Study the drawing (mm; zero at the part's minimum x, y, z) and answer. A direction names the side the tool comes from. Coordinates: 2 decimals unless noted, no trailing zeros. Loops run counter-clockwise (first coordinate to the right, second up) from the corner with the lowest first, then second, coordinate; pieces in that order, holes last. Notation, with made-up numbers: (-26.75, -5) - (-9.75, -5) arc R24 ccw to (-9.75, 28) - close; hole circle Ø3 at (87.5, 3.5). An arc over 180 degrees is marked (long way). Use CSV: the item, a comma, the result in double quotes.
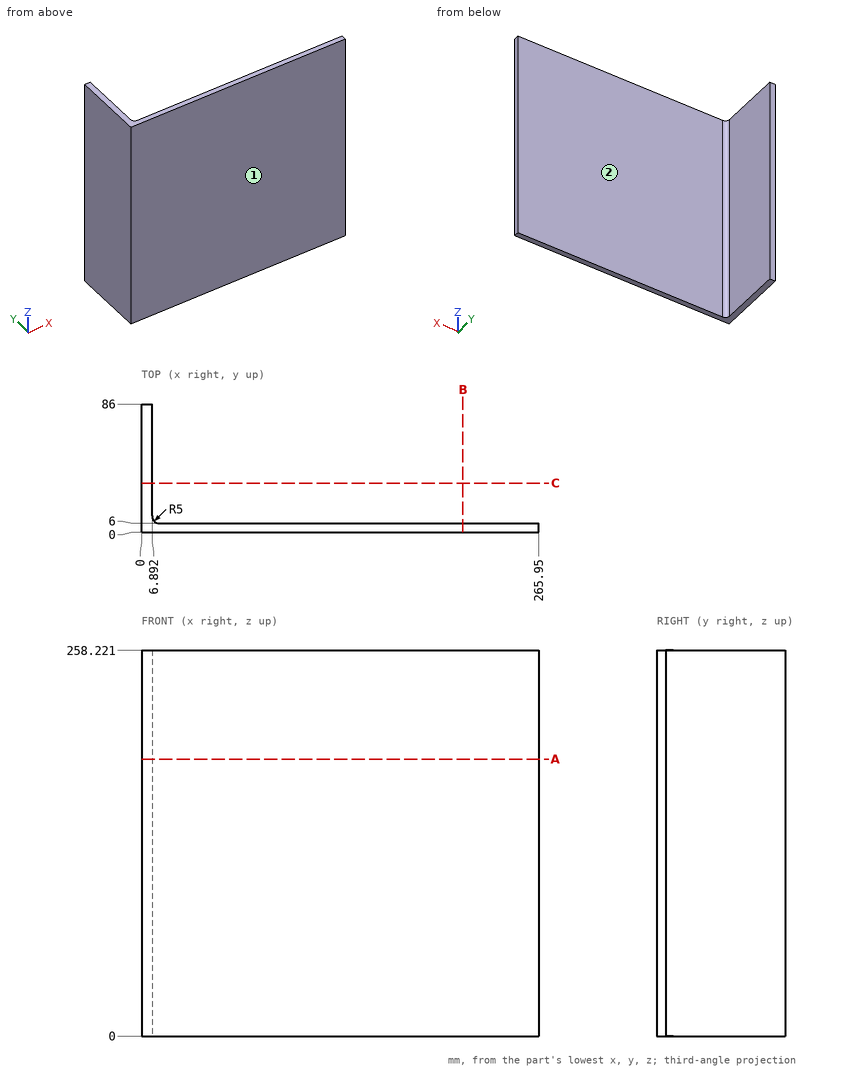
Q1. Given P1, Ø12, axis at y = 35, z = 41.5, coming from the +X side; P2, Ø5, axis at x = 149, z = 41, coming from the +Y side, each flat-ended and moving along its own axis, determine where each tip first touches the part or whether it passes through.
Reported:
P1,"stops at x = 6.89"
P2,"stops at y = 6"
Q2. The part is cut by section C-C on y = 33. Determine the outline of the cut face in (x, z), and give its area (3 significant figures).
Reported:
outline,"(0, 0) - (6.89, 0) - (6.89, 258.22) - (0, 258.22) - close"
area,"1,780 mm²"
Q3. The part is cut by section A-A on z = 185.5. Determine the outline of the cut face in (x, y).
Reported:
outline,"(0, 0) - (265.95, 0) - (265.95, 6) - (11.89, 6) arc R5 cw to (6.89, 11) - (6.89, 86) - (0, 86) - close"
Q4. The part is cut by section B-B on x = 215. Determine the outline of the cut face in (y, z).
Reported:
outline,"(0, 0) - (6, 0) - (6, 258.22) - (0, 258.22) - close"
Q5. Find the intervals of material crossed by probe 1 along Y at (x, z) = (200.5, 182); probe 2 along X at (y, z) = (18, 143.5); probe 3 along X at (y, z) = (9, 151.5), in increasing order. Write a range as [from, to].
Reported:
probe 1,"y = [0, 6]"
probe 2,"x = [0, 6.89]"
probe 3,"x = [0, 7.31]"
Q6. A tool of negligible diameter and unlimited length cuts with its end or side. For the marked faces 1 and 2, from which of +Z, -Z, +X, -X, +Y, -Y can it reach the whole face along a straight path? Write none if from no direction.
Reported:
face 1,"+Z, -Z, +X, -X, -Y"
face 2,"+Z, -Z, +X, +Y"
